Model file for the job. Use its own axes, mm. A direction names the side the tool comes from. Give positions to 0.01 mm unless a question says otherwise; leave off trailing zeros. Write each loop counter-clockwise with the first axis right and the second up, starting at its lowest first coordinate (ties: lowest second). Pieces come first, ordered by that corner, then holes.
```python
from build123d import *

# Parameters (mm, degrees)
SKETCH3_R           = 2
CUT_EXTRUDE1_DEPTH  = 14.8
CUT_EXTRUDE2_START  = -2
SKETCH4_R           = 4.05
CUT_EXTRUDE2_DEPTH  = 12.8
BOSS_EXTRUDE1_START = 3
SKETCH5_R           = 12
SKETCH5_R_2         = 2
BOSS_EXTRUDE1_DEPTH = 3


with BuildPart() as part:
    # Sketch2 → Revolve1 (revolve)
    with BuildSketch(Plane(origin=(0, 0, 0), x_dir=(1, 0, 0), z_dir=(0, 1, 0))):
        Polygon((-7.7, 12), (-7.7, 0), (-7.1, 0), (7.1, 0), (7.1, 12), (6.6, 12), (4.6, 10), (-4.6, 10), (-6.6, 12), (-7.1, 12), align=None)
    revolve(axis=Axis((7.1, 0, 0), (-1, 0, 0)))

    # Sketch3 → Cut-Extrude1 (cut)
    with BuildSketch(Plane.ZY.offset(7.7)):
        Circle(SKETCH3_R)
    extrude(amount=-CUT_EXTRUDE1_DEPTH, mode=Mode.SUBTRACT)

    # Sketch4 → Cut-Extrude2 (cut)
    with BuildSketch(Plane.ZY.offset(7.7).offset(CUT_EXTRUDE2_START)):
        Circle(SKETCH4_R)
    extrude(amount=-CUT_EXTRUDE2_DEPTH, mode=Mode.SUBTRACT)

    # Sketch5 → Boss-Extrude1 (add)
    with BuildSketch(Plane.ZY.offset(7.7).offset(BOSS_EXTRUDE1_START)):
        with Locations(Location((0, 0, 0), (0, 0, 180))):
            Circle(SKETCH5_R)
        Circle(SKETCH5_R_2, mode=Mode.SUBTRACT)
    extrude(amount=-BOSS_EXTRUDE1_DEPTH)


solid = part.part
```
1. Which spindle directions (+Z, -Z, +X, -X, +Y, -Y) get a long thin tool onto all of the face, cutting with end or side? Do faces 1 (the cylindrical face through (-0.06, 9.76, 2.17)), 2 (the cylindrical face through (0.61, -3.954, -0.878)), 3 (the cylindrical face through (-8.679, -3.604, -11.446)). Say none if no direction does.
Calculated:
face 1: none
face 2: +X
face 3: +X, -X
2. Slice it at C-C, the plane x = -4. Write the cut outline in (y, z), and give its area (3 significant figures).
Calculated:
outline: circle Ø20 at (0, 0); hole circle Ø8.1 at (0, 0)
area: 263 mm2
3. Pull direction Z, two halves, no side cores. Call faces 4 (the flat face through (-5.7, -1, -2)), 5 (the flat face through (-10.7, -0.2, -2.5)), 6 (the conical face through (-4.725, 9.884, 2.195)): +Z half, -Z half, draft (parallel to the pull), parting line (faces both ways), or undercut.
Calculated:
face 4: undercut
face 5: draft
face 6: parting line
4. Pin check, flat tips, straight feed: P1, Ø6, axis at x = -2.5, y = -5, coming from the -Z side; P2, Ø1, axis at x = 5.5, y = 1, coming from the -Z side; P3, Ø1, axis at x = -2.5, z = -2, coming from the +Y side. Stop position of each tip, or through.
Calculated:
P1: stops at z = -9.96
P2: stops at z = -11.36
P3: stops at y = 9.89
5. Probe probe 1 along Y at (x, z) = (0, 0); probe 2 along Y at (x, z) = (-9.7, 0); probe 3 along X at (y, z) = (-10, 1.25). List the from-to ranges inside material, lowest first.
Calculated:
probe 1: y = -10 to -4.05, 4.05 to 10
probe 2: y = -12 to -2, 2 to 12
probe 3: x = -10.7 to -4.68, 4.68 to 7.1
6. Slice it at A-A, the plane y = 0. Write the cut outline in (x, z), and give its area (3 significant figures).
Calculated:
outline: (-10.7, -12) - (-6.6, -12) - (-4.6, -10) - (4.6, -10) - (6.6, -12) - (7.1, -12) - (7.1, -4.05) - (-5.7, -4.05) - (-5.7, -2) - (-10.7, -2) - close; (-10.7, 2) - (-5.7, 2) - (-5.7, 4.05) - (7.1, 4.05) - (7.1, 12) - (6.6, 12) - (4.6, 10) - (-4.6, 10) - (-6.6, 12) - (-10.7, 12) - close
area: 259 mm2
